Could you check a few things on this model? Use its own coordinates, in mm. Coordinates: 2 decimals unless noted, no trailing zeros. Loops run counter-clockwise (first coordinate to the right, second up) from the corner with the lowest first, then second, coordinate; pieces in that order, holes last.
Autodesk Inventor part; units mm, degrees
ref_plane "YZ Plane" through (0, 0, 0) normal (1, 0, 0) x (0, 1, 0)
ref_plane "XZ Plane" through (0, 0, 0) normal (0, 1, 0) x (-1, 0, 0)
ref_plane "XY Plane" through (0, 0, 0) normal (0, 0, 1) x (1, 0, 0)
sketch "Sketch1" plane through (0, 0, 0) normal (0, 1, 0) x (-1, 0, 0)
  circle A0 centre (0, 0) radius 45
  line L0 (0, 0) -> (0, -40.64)
  line L1 (0, -40.64) -> (-8.89, -40.64)
  circle A1 centre (-8.89, -40.64) radius 1.5
  circle A2 centre (40.64, -8.89) radius 1.5
  circle A3 centre (8.89, 40.64) radius 1.5
  circle A4 centre (-40.64, 8.89) radius 1.5
  dimension "d0" = 90
  dimension "d1" = 40.64
  dimension "d2" = 8.89
  dimension "d3" = 3
  dimension "d6" = 360
extrude "Extrusion1" add sketch "Sketch1" along normal blind 1.5
sketch "Sketch2" plane through (0, 1.5, 0) normal (0, 1, 0) x (1, 0, 0)
  point P0 (0, 0)
properties part number "Light Sensor"
(1) I need wall thicknesses on probe 1 along Z at (x, y) = (40.64, 1.1); probe 2 along Z at (x, y) = (8.89, 1.1); probe 3 along Z at (x, y) = (-36, 0.1). Which ranges of each line are inside material? Lowest first, please.
Answers:
probe 1: z = -19.32 to 7.39, 10.39 to 19.32
probe 2: z = -44.11 to -42.14, -39.14 to 44.11
probe 3: z = -27 to 27
(2) Imagine slicing it at D-D, the plane x = -14.5. Write out the boundary of the cut face in (y, z), and give its area (3 significant figures).
Answers:
outline: (0, -42.6) - (1.5, -42.6) - (1.5, 42.6) - (0, 42.6) - close
area: 128 mm2
(3) We'd pull the mould along Z, two halves only. Please class faces 1 (the face through (-8.565, 0.74, 42.104)), 2 (the face through (1, 0, 1)), 3 (the face through (-20.765, 0.74, 39.923)): +Z half, -Z half, draft (parallel to the pull), parting line (faces both ways), or undercut.
Answers:
face 1: undercut
face 2: draft
face 3: parting line
(4) Imagine slicing it at C-C, the plane z = -40.64. Write out the boundary of the cut face in (x, y).
Answers:
outline: (-19.32, 0) - (7.39, 0) - (7.39, 1.5) - (-19.32, 1.5) - close; (10.39, 0) - (19.32, 0) - (19.32, 1.5) - (10.39, 1.5) - close
(5) For pin 1 (1 mm diameter, centred on x = 0.5, z = -8.5, fed in from -Y); pin 2 (2.5 mm diameter, centred on x = 40.64, z = 8.89, fed in from -Y), each with a flat end and sliding along its axis, tell me the tip position at first contact or that it passes through.
Answers:
pin 1: stops at y = 0
pin 2: passes through
(6) Imagine slicing it at A-A, the plane y = 0.45. Write out the boundary of the cut face in (x, z).
Answers:
outline: circle Ø90 at (0, 0); hole circle Ø3 at (-40.64, -8.89); hole circle Ø3 at (-8.89, 40.64); hole circle Ø3 at (8.89, -40.64); hole circle Ø3 at (40.64, 8.89)
(7) Imagine slicing it at B-B, the plane x = 8.89. Write out the boundary of the cut face in (y, z), and give its area (3 significant figures).
Answers:
outline: (0, -44.11) - (1.5, -44.11) - (1.5, -42.14) - (0, -42.14) - close; (0, -39.14) - (1.5, -39.14) - (1.5, 44.11) - (0, 44.11) - close
area: 128 mm2
